For this review, use the dimensioned drawing (mm, ordinates from the lowest corner) and the shaded views. Round coordinates to 2 decimals unless told otherwise and drop trailing zeros. Loops run counter-clockwise (first coordinate to the right, second up) from the corner with the lowest first, then second, coordinate; pieces in that order, holes last. Notation, with made-up numbers: M -21.5,-27.75 L 25.5,-27.75 A22 cw 25.5,-5.75 Z; hole C 22,-35 d9. An arc over 180 degrees is marked long. Answer as a JSON object with one key per item and string values. Group by question number.
Item 1: To check wall thickness, follow line 1 (Z direction, x = 65, y = 2); line 2 (Z direction, x = 43.5, y = 3); line 3 (X direction, y = 1.25, z = 5). State the ranges of each line that lie inside material, in increasing order.
Item 2: Insertion check: P1, Ø5, axis at x = 27, z = 58, coming from the -Y side. The pin has a flat end and moves straight along its axis. Give the tip position at first contact, or say it passes through.
Item 3: Consider section A-A (x = 59). Give the boundary of the cut face in (y, z).
Item 4: Consider section B-B (z = 29.5). Give the boundary of the cut face in (x, y).
Item 5: The part is to be moulded in two halves that separate along Z. For the marked faces 1, 2, 3 and 4, say which applies: +Z half, -Z half, draft (parallel to the pull), parting line (faces both ways), or undercut.
Item 6: Consider section C-C (z = 7). Give the boundary of the cut face in (x, y).
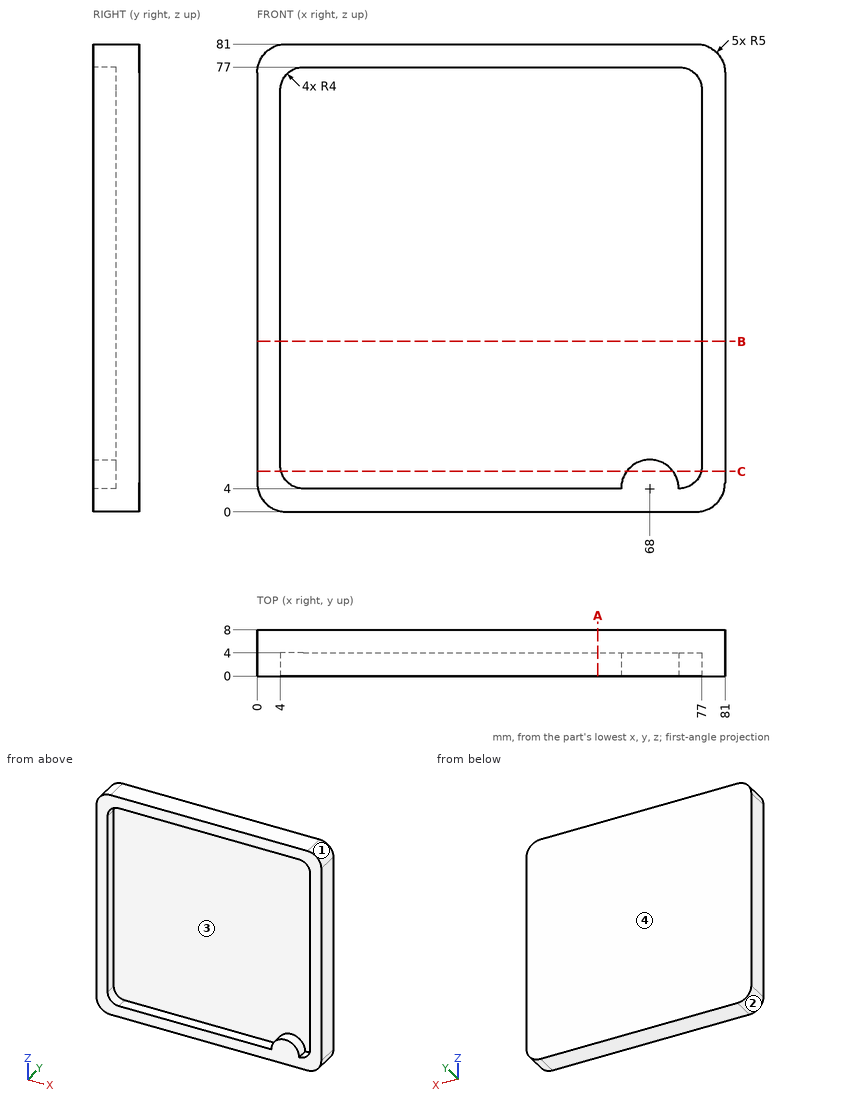
Geometry results:
{
 "1": {"line 1": "z = 0 to 8, 77 to 81", "line 2": "z = 0 to 4, 77 to 81", "line 3": "x = 0 to 5.35, 63.1 to 72.9, 75.65 to 81"},
 "2": {"P1": "stops at y = 4"},
 "3": {"outline": "M 0,0 L 8,0 L 8,81 L 0,81 L 0,77 L 4,77 L 4,4 L 0,4 Z"},
 "4": {"outline": "M 0,0 L 4,0 L 4,4 L 77,4 L 77,0 L 81,0 L 81,8 L 0,8 Z"},
 "5": {"face 1": "+Z half", "face 2": "-Z half", "face 3": "undercut", "face 4": "draft"},
 "6": {"outline": "M 0,0 L 4.13,0 L 4.13,4 L 64,4 L 64,0 L 72,0 L 72,4 L 76.87,4 L 76.87,0 L 81,0 L 81,8 L 0,8 Z"}
}
